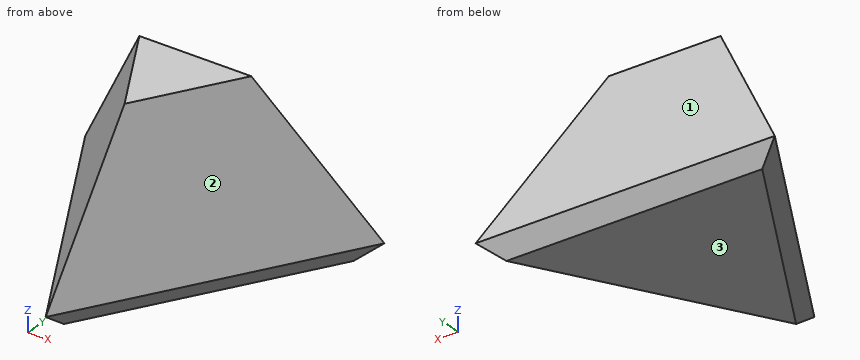
from build123d import *

# Parameters (mm, degrees)
F1_DEPTH = 87.5
F1_TAPER = 20
F2_SIZE  = 10


with BuildPart() as f1:
    # F0 (on Top) → F1 (new body)
    with BuildSketch(Plane.XY):
        Polygon((84.5943443278, 48.8405674696), (-84.5943443278, 48.8405674696), (0, -97.6811349392), align=None)
    extrude(amount=F1_DEPTH, taper=F1_TAPER)

    # F2
    f2_edges = [f1.edges().sort_by_distance(p)[0] for p in [
        (42.297172, -24.420284, 0),
        (-42.297172, -24.420284, 0),
        (0, 48.840567, 0),
    ]]
    chamfer(f2_edges, length=F2_SIZE)


solid = f1.part
Design review of the part built by this model. Coordinates are the model's own, in mm. Face numbers are marked on the shaded views. Round coordinates to 2 decimals unless told otherwise and drop trailing zeros. Write each loop counter-clockwise with the first axis right and the second up, starting at its lowest first coordinate (ties: lowest second). Pieces come first, ordered by that corner, then holes. Notation, with made-up numbers: (26, 56.5) - (41, 56.5) arc R31 ccw to (41, 87.5) - close; hole circle Ø11 at (-33.75, 72.5). An arc over 180 degrees is marked (long way). Use a Markdown table: item, result. Add a question column.
1. We need section B-B (x = -24). State the section outline as (y, z) points, then the cut area to 3 significant figures.
2. Clearance check with flat-ended pins moving along their axes: pin 1 (12 mm diameter, centred on x = -8, z = 43, fed in from +Y); pin 2 (2 mm diameter, centred on y = -1.5, z = 44, fed in from +X); pin 3 (2 mm diameter, centred on y = 22.5, z = 64, fed in from -X). State where each tip first meets the part, or that it passes through.
3. We need section C-C (z = 40.5). State the section outline as (x, y) points.
4. Wall thickness on probe 1 along Y at (x, z) = (4, 10); probe 2 along Y at (x, z) = (16.5, 56.5); probe 3 along X at (y, z) = (4.5, 52): over which ranges is each line inside the solid? List them lowest first.
5. We need section A-A (y = -36.5). State the section outline as (x, z) points.
6. We need section D-D (x = 38). State the section outline as (y, z) points.
7. Mouldability with a two-part tool opening along Y and no side actions: class the marked faces 1, 2 and 3 as +Y half, -Y half, draft (parallel to the pull), parting line (faces both ways), or undercut.
Output:
| question | item | result |
|---|---|---|
| 1 | outline | (-49.27, 9.4) - (-36.11, 0) - (38.84, 0) - (45.42, 9.4) - (16.99, 87.5) - (7.58, 87.5) - close |
| 1 | area | 4,860 mm2 |
| 2 | pin 1 | stops at y = 35.37 |
| 2 | pin 2 | stops at x = 37.75 |
| 2 | pin 3 | stops at x = -43.2 |
| 3 | outline | (-59.06, 34.1) - (0, -68.2) - (59.06, 34.1) - close |
| 4 | probe 1 | y = -83.47 to 45.2 |
| 4 | probe 2 | y = -27.97 to 28.28 |
| 4 | probe 3 | x = -37.14 to 37.14 |
| 5 | outline | (-31.37, 9.4) - (-23.78, 0) - (23.78, 0) - (31.37, 9.4) - (0, 84.05) - close |
| 6 | outline | (-25.02, 9.4) - (-11.86, 0) - (38.84, 0) - (45.42, 9.4) - (21.94, 73.91) - close |
| 7 | face 1 | +Y half |
| 7 | face 2 | -Y half |
| 7 | face 3 | draft |
